Part print with two shaded views. Sizes in mm from the minimum x, y, z corner. Round coordinates to 2 decimals unless told otherwise and drop trailing zeros. Write each loop counter-clockwise with the first axis right and the second up, starting at its lowest first coordinate (ties: lowest second). Pieces come first, ordered by that corner, then holes. Notation, with made-up numbers: (78.5, -35.5) -> (86.5, -35.5) arc R17 ccw to (86.5, -4.5) -> close; hole circle Ø8 at (-22.75, 6.5). An arc over 180 degrees is marked (long way). Put each result on its own line as item: value. Start each with the question number.
1. Saw through at C-C on z = 67.5. List the corners of the cut face in (x, y), and give its area (3 significant figures).
2. Saw through at A-A on y = 2.35. List the corners of the cut face in (x, z), and give its area (3 significant figures).
3. Saw through at B-B on x = 79.5. List the corners of the cut face in (y, z), and give its area (3 significant figures).
4. Flat gauge pins, fed straight in: P1, Ø3, axis at x = 17, z = 18.32, coming from the -Y side; P2, Ø1.5, axis at y = 2, z = 55, coming from the +X side. Where does each tip first touch, or does it go through?
5. Drill centre lines: line 1 (X direction, y = 2.15, z = 95); line 2 (Z direction, x = 86.5, y = 0.9). Where is each one in solid material? Low to high. Write a range as from..to.
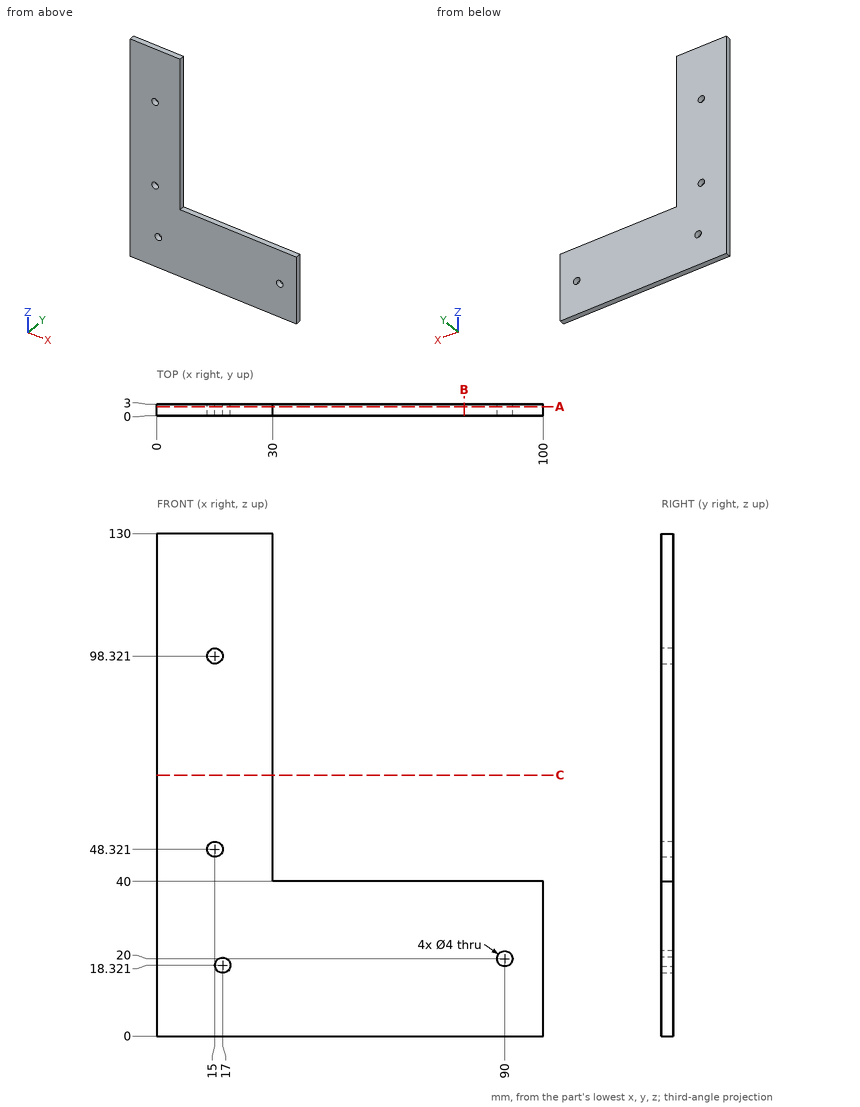
Return value:
1. outline: (0, 0) -> (30, 0) -> (30, 3) -> (0, 3) -> close
1. area: 90.0 mm^2
2. outline: (0, 0) -> (100, 0) -> (100, 40) -> (30, 40) -> (30, 130) -> (0, 130) -> close; hole circle Ø4 at (15, 48.32); hole circle Ø4 at (15, 98.32); hole circle Ø4 at (17, 18.32); hole circle Ø4 at (90, 20)
2. area: 6,650 mm^2
3. outline: (0, 0) -> (3, 0) -> (3, 40) -> (0, 40) -> close
3. area: 120 mm^2
4. P1: passes through
4. P2: stops at x = 30
5. line 1: x = 0..30
5. line 2: z = 0..40
